Read the model definition and answer for the solid it produces. Units are mm, in the model's axes. Coordinates: 2 decimals unless noted, no trailing zeros. Loops run counter-clockwise (first coordinate to the right, second up) from the corner with the lowest first, then second, coordinate; pieces in that order, holes last. Notation, with made-up numbers: (89.25, 31) -> (102.25, 31) arc R23 ccw to (102.25, 53) -> close; hole circle Ø10 at (74, 54.25). An arc over 180 degrees is marked (long way). Answer in a Markdown table with one row per item.
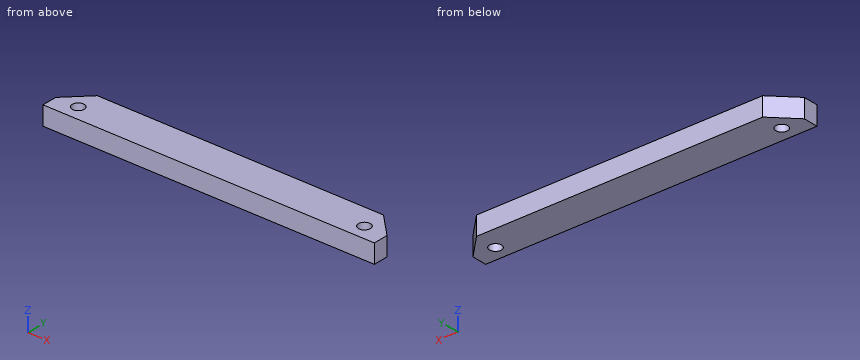
```python
from build123d import *

# Parameters (mm, degrees)
DODANIE_WYCI_GNI_CIE1_DEPTH = 5
SZKIC2_R                    = 1.6
WYTNIJ_WYCI_GNI_CIE1_DEPTH  = 46.495164578


with BuildPart() as part:
    # Szkic1 → Dodanie-wyciągnięcie1 (new body)
    with BuildSketch(Plane.XY):
        Polygon((-44.1, 0), (44.1, 0), (44.1, 4), (38.1, 10), (-38.1, 10), (-44.1, 4), align=None)
    extrude(amount=DODANIE_WYCI_GNI_CIE1_DEPTH)

    # Szkic2 → Wytnij-wyciągnięcie1 (cut, through all)
    with BuildSketch(Plane.XY.offset(5)):
        with Locations((-38.1, 4)):
            Circle(SZKIC2_R)
        with Locations(Location((38.1, 4, 0), (0, 0, 180))):
            Circle(SZKIC2_R)
    extrude(amount=-WYTNIJ_WYCI_GNI_CIE1_DEPTH, mode=Mode.SUBTRACT)


solid = part.part
```
1. Find the intervals of material crossed by probe 1 along Y at (x, z) = (38.1, 2.8); probe 2 along X at (y, z) = (4.75, 1.6); probe 3 along X at (y, z) = (4.25, 4.85), in increasing order.
A:
| item | result |
|---|---|
| probe 1 | y = 0 to 2.4, 5.6 to 10 |
| probe 2 | x = -43.35 to -39.51, -36.69 to 36.69, 39.51 to 43.35 |
| probe 3 | x = -43.85 to -39.68, -36.52 to 36.52, 39.68 to 43.85 |
2. A cutting plane is placed at A-A on z = 3.95. Give the vertices of the cut face in (x, y).
A:
| item | result |
|---|---|
| outline | (-44.1, 0) -> (44.1, 0) -> (44.1, 4) -> (38.1, 10) -> (-38.1, 10) -> (-44.1, 4) -> close; hole circle Ø3.2 at (-38.1, 4); hole circle Ø3.2 at (38.1, 4) |
3. A cutting plane is placed at B-B on y = 7.5. Give the vertices of the cut face in (x, z).
A:
| item | result |
|---|---|
| outline | (-40.6, 0) -> (40.6, 0) -> (40.6, 5) -> (-40.6, 5) -> close |
4. Given pin 1 Ø3 at (x, z) = (-26, 3.5) entering from -Y, flat-ended and moving along its own axis, determine where the tip first touches the part or whether it passes through.
A:
| item | result |
|---|---|
| pin 1 | stops at y = 0 |
